from build123d import *

# Parameters (mm, degrees)
SKETCH_1_W      = 53
SKETCH_1_H      = 53
SKETCH_1_R      = 21.5
EXTRUDE_1_DEPTH = 7
EXTRUDE_START   = 3
SKETCH_2_W      = 53
SKETCH_2_H      = 53
SKETCH_2_R      = 0.8
SKETCH_2_R_2    = 9
EXTRUDE_2_DEPTH = 3


with BuildPart() as part:
    # 草图1 → 凸台-拉伸1 (new body)
    with BuildSketch(Plane(origin=(0, 0, 0), x_dir=(1, 0, 0), z_dir=(0, 1, 0))):
        Rectangle(SKETCH_1_W, SKETCH_1_H)
        with Locations(Location((0, 0, 0), (0, 0, 270))):
            Circle(SKETCH_1_R, mode=Mode.SUBTRACT)
    extrude(amount=EXTRUDE_1_DEPTH)

    # 草图2 → 凸台-拉伸2 (add)
    with BuildSketch(Plane.XZ.offset(EXTRUDE_START)):
        Rectangle(SKETCH_2_W, SKETCH_2_H)
        with Locations(Location((-13, -7.505553499, 0), (0, 0, 270))):
            Circle(SKETCH_2_R, mode=Mode.SUBTRACT)
        with Locations(Location((0, 15.011106999, 0), (0, 0, 270))):
            Circle(SKETCH_2_R, mode=Mode.SUBTRACT)
        with Locations(Location((13, -7.505553499, 0), (0, 0, 270))):
            Circle(SKETCH_2_R, mode=Mode.SUBTRACT)
        with Locations(Location((0, 0, 0), (0, 0, 270))):
            Circle(SKETCH_2_R_2, mode=Mode.SUBTRACT)
        with BuildLine():
            Line((-6, -20.645822822), (-6, -10.645822822))
            Line((-6, -10.645822822), (6, -10.645822822))
            Line((6, -10.645822822), (6, -20.645822822))
            ThreePointArc((6, -20.645822822), (0, -21.5), (-6, -20.645822822))
        make_face(mode=Mode.SUBTRACT)
    extrude(amount=-EXTRUDE_2_DEPTH)


solid = part.part
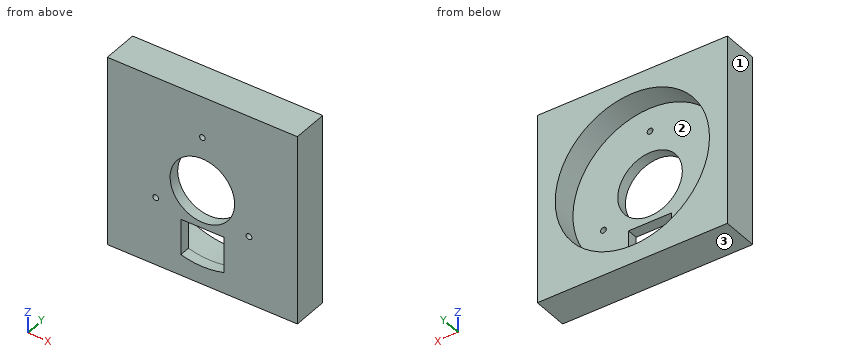
Source: CAD feature listing. Evaluate the final solid. Frame: model axes, mm. Face numbers are marked on the shaded views. Coordinates: 2 decimals unless noted, no trailing zeros. Order: outer loops, then holes, each group sorted by start corner. A loop starts at its lowest first (then second) coordinate and runs counter-clockwise, first axis right, second up. Notation, with made-up numbers: M 22,40.5 L 28,40.5 A30 ccw 28,75.5 Z; hole C -36.75,-36 d2. An arc over 180 degrees is marked long. Write each question's results on one line, items separated by ' | '. Start each with the question number.
1. Section C-C, the plane x = 0. Return the cut outline in (y, z).
2. Section D-D, the plane y = 5.75. Return the cut outline in (x, z), then the cut area to 3 significant figures.
3. Section A-A, the plane z = 0. Return the cut outline in (x, y).
4. Section B-B, the plane y = -1. Return the cut outline in (x, z), then the cut area to 3 significant figures.
5. Draft query along Z for the marked faces 1, 2 and 3. Return one class per face: +Z half, -Z half, draft (parallel to the pull), parting line (faces both ways), or undercut.
6. Pin query (flat end, axial travel): pin 1 (2.5 mm diameter, centred on x = 13, z = -7.51, fed in from -Y); pin 2 (1 mm diameter, centred on x = 0, z = 15.01, fed in from +Y); pin 3 (6 mm diameter, centred on x = 9, z = -7.5, fed in from +Y). Return the tip coordinate at first contact, or that it passes through.
7. Material intervals for L1, parallel to Z at x = 0, y = 4; L2, parallel to X at y = -2, z = -7.5, sorted ascending.
Solution:
1) outline: M -3,-26.5 L 7,-26.5 L 7,-21.5 L -3,-21.5 Z; M -3,-10.65 L 0,-10.65 L 0,-9 L -3,-9 Z; M -3,9 L 0,9 L 0,14.21 L -3,14.21 Z; M -3,15.81 L 0,15.81 L 0,21.5 L 7,21.5 L 7,26.5 L -3,26.5 Z
2) outline: M -26.5,-26.5 L 26.5,-26.5 L 26.5,26.5 L -26.5,26.5 Z; hole C 0,0 d43 | area: 1,360 mm²
3) outline: M -26.5,-3 L -9,-3 L -9,0 L -21.5,0 L -21.5,7 L -26.5,7 Z; M 9,-3 L 26.5,-3 L 26.5,7 L 21.5,7 L 21.5,0 L 9,0 Z
4) outline: M -26.5,-26.5 L 26.5,-26.5 L 26.5,26.5 L -26.5,26.5 Z; hole C -13,-7.51 d1.6; hole C 0,0 d18; hole M -6,-20.65 A21.5 ccw 6,-20.65 L 6,-10.65 L -6,-10.65 Z; hole C 0,15.01 d1.6; hole C 13,-7.51 d1.6 | area: 2,420 mm²
5) face 1: draft | face 2: undercut | face 3: -Z half
6) pin 1: y = -3 | pin 2: through | pin 3: y = 0
7) L1: -26.5 to -21.5, 21.5 to 26.5 | L2: -26.5 to -13.8, -12.2 to -4.97, 4.97 to 12.2, 13.8 to 26.5
